from build123d import *

# Parameters (mm, degrees)
F0_W     = 149.531708
F0_H     = 150.427163
F1_DEPTH = 4.8
F2_W     = 75.19953
F2_H     = 30.355446
F3_DEPTH = 33
F5_DEPTH = 149.5


with BuildPart() as f1:
    # F0 (on Front) → F1 (new body)
    with BuildSketch(Plane.XZ):
        with Locations((0.433676, -0.481956)):
            Rectangle(F0_W, F0_H)
    extrude(amount=F1_DEPTH)

    # F2 (on face) → F3 (cut)
    with BuildSketch(Plane.XZ.offset(4.8)):
        with Locations((37.599765, 31.643964)):
            Rectangle(F2_W, F2_H)
    extrude(amount=-F3_DEPTH, mode=Mode.SUBTRACT)

    # F4 (on face) → F5 (join)
    with BuildSketch(Plane.YZ.offset(75.19953)):
        with BuildLine():
            Line((0, -56.370427), (0, -63.030267))
            Line((0, -63.030267), (121.53174, -45.979694))
            Line((121.53174, -45.979694), (136.657913, -38.343303))
            Line((136.657913, -38.343303), (136.117308, -35.507916))
            ThreePointArc((136.117308, -35.507916), (134.016588, -32.309223), (130.269337, -31.53284))
            Line((130.269337, -31.53284), (0, -56.370427))
        make_face()
        with BuildLine():
            Line((-15.475349, -63.457762), (-15.475349, -65.201417))
            Line((-15.475349, -65.201417), (-4.8, -63.703694))
            Line((-4.8, -63.703694), (-4.8, -57.285611))
            Line((-4.8, -57.285611), (-11.411796, -58.546238))
            ThreePointArc((-11.411796, -58.546238), (-14.327766, -60.270462), (-15.475349, -63.457762))
        make_face()
    extrude(amount=-F5_DEPTH)


solid = f1.part
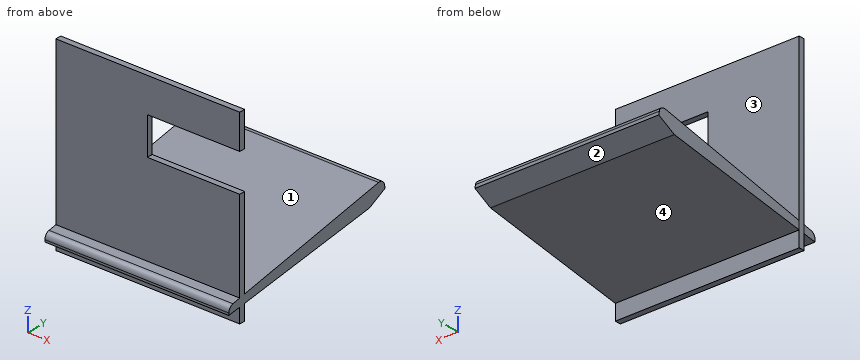
Geometry: final body of the model. Coordinates: model frame, mm. Face numbers are marked on the shaded views. A direction names the side the tool comes from. Coordinates: 2 decimals unless noted, no trailing zeros. Order: outer loops, then holes, each group sorted by start corner. A loop starts at its lowest first (then second) coordinate and runs counter-clockwise, first axis right, second up. Notation, with made-up numbers: (-1.5, -5) - (23.5, -5) arc R17 ccw to (23.5, 1) - close; hole circle Ø6 at (-32, 13.25). An arc over 180 degrees is marked (long way). Use one line per item in the form item = value.
1) Section D-D (z = -28). Return loops of the section in (x, y).
Solutions:
outline = (-74.33, -4.8) - (75.2, -4.8) - (75.2, 0) - (-74.33, 0) - close
2) Mould query, pull axis Y, two halves, no side actions, for the marked faces 1 and 2. Classes: +Y half, -Y half, draft (parallel to the pull), parting line (faces both ways), or undercut.
Solutions:
face_1 = undercut
face_2 = +Y half
3) Section C-C (x = 52.5). Return loops of the section in (y, z).
Solutions:
outline = (-15.48, -65.2) - (-4.8, -63.7) - (-4.8, -75.7) - (0, -75.7) - (0, -63.03) - (121.53, -45.98) - (136.66, -38.34) - (136.12, -35.51) arc R5 ccw to (130.27, -31.53) - (0, -56.37) - (0, 16.47) - (-4.8, 16.47) - (-4.8, -57.29) - (-11.41, -58.55) arc R5 ccw to (-15.48, -63.46) - close; (-4.8, 46.82) - (0, 46.82) - (0, 74.73) - (-4.8, 74.73) - close
4) Section B-B (x = -62.5). Return loops of the section in (y, z).
Solutions:
outline = (-15.48, -65.2) - (-4.8, -63.7) - (-4.8, -75.7) - (0, -75.7) - (0, -63.03) - (121.53, -45.98) - (136.66, -38.34) - (136.12, -35.51) arc R5 ccw to (130.27, -31.53) - (0, -56.37) - (0, 74.73) - (-4.8, 74.73) - (-4.8, -57.29) - (-11.41, -58.55) arc R5 ccw to (-15.48, -63.46) - close
5) Section A-A (z = -49). Return loops of the section in (x, y), then the cut area to 3 significant figures.
Solutions:
outline = (-74.33, -4.8) - (75.2, -4.8) - (75.2, 0) - (-74.33, 0) - close; (-74.3, 38.66) - (75.2, 38.66) - (75.2, 100) - (-74.3, 100) - close
area = 9,890 mm^2
6) Pin query (flat end, axial travel): pin 1 (2.5 mm diameter, centred on y = -10.5, z = -60.5, fed in from -X); pin 2 (10 mm diameter, centred on x = 10, y = 69.5, fed in from -Z); pin 3 (10 mm diameter, centred on x = 30, y = 74, fed in from -Z). Return the tip coordinate at first contact, or that it passes through.
Solutions:
pin_1 = -74.3
pin_2 = -53.98
pin_3 = -53.35
7) Ray query, L1, parallel to Y at x = 46, z = 53; L2, parallel to Z at x = 62.5, y = 104.5; L3, parallel to Z at x = -37, y = 105. Return the intervals inside material, ascending.
Solutions:
L1 = -4.8 to 0
L2 = -48.37 to -36.45
L3 = -48.3 to -36.35
8) Set-up query: the marked faces 3 and 4. Return all of +Z, -Z, +X, -X, +Y, -Y with unobstructed straight access to the full face (end or side cutting, diameter ignored); none if empty.
Solutions:
face_3 = +X, -X
face_4 = -Z, +X, -X, +Y
